Verification items for the finished model (mm, model axes). Give positions to 0.01 mm unless a question says otherwise; leave off trailing zeros. Write each loop counter-clockwise with the first axis right and the second up, starting at its lowest first coordinate (ties: lowest second). Pieces come first, ordered by that corner, then holes. Notation, with made-up numbers: (26, 60.5) -> (47, 60.5) arc R22 ccw to (47, 68.5) -> close; hole circle Ø5 at (27, -12.75). An arc over 180 degrees is marked (long way). Use one line per item in the form item = value. Start each with the question number.
(1) Section check B-B, the plane x = 0. Record the cut outline in (y, z) (1 decimal).
(2) Section check C-C, the plane y = -16.51. State how many separate pieces and enclosed holes the cut face has, plus the area to 3 significant figures.
(3) Section check A-A, the plane z = -8.89. Record the cut outline in (x, y) (3 decimals).
(4) Scan lines: L1, parallel to X at y = -7.5, z = -8.89; L2, parallel to X at y = -12.5, z = -4; L3, parallel to X at y = -10.5, z = -6.5. Record each from-to range of solid material in increasing order.
(5) Depth check by flat-ended pin: pin 1 Ø4 at (x, y) = (122.95, -16.51) entering from +Z; pin 2 Ø3 at (x, y) = (120.5, -15) entering from +Z. Enter the tip coordinate at first touch or a pass-through.
from build123d import *

# Parameters (mm, degrees)
SKETCH1_W           = 266.7
SKETCH1_H           = 17.78
SKETCH1_R           = 3.96875
BOSS_EXTRUDE1_DEPTH = 33.02
SKETCH2_R           = 3.175
CUT_EXTRUDE1_DEPTH  = 17.78
SKETCH3_R           = 4.7625
CUT_EXTRUDE2_DEPTH  = 4.7752


with BuildPart() as part:
    # Sketch1 → Boss-Extrude1 (new body)
    with BuildSketch(Plane(origin=(0, 0, 0), x_dir=(1, 0, 0), z_dir=(0, 1, 0))):
        with Locations((0, 8.89)):
            Rectangle(SKETCH1_W, SKETCH1_H)
        with Locations(Location((108.585, 8.89, 0), (0, 0, 270))):
            Circle(SKETCH1_R, mode=Mode.SUBTRACT)
        with Locations(Location((36.195, 8.89, 0), (0, 0, 270))):
            Circle(SKETCH1_R, mode=Mode.SUBTRACT)
        with Locations(Location((-36.195, 8.89, 0), (0, 0, 270))):
            Circle(SKETCH1_R, mode=Mode.SUBTRACT)
        with Locations(Location((-108.585, 8.89, 0), (0, 0, 270))):
            Circle(SKETCH1_R, mode=Mode.SUBTRACT)
    extrude(amount=-BOSS_EXTRUDE1_DEPTH)

    # Sketch2 → Cut-Extrude1 (cut)
    with BuildSketch(Plane.XY):
        with Locations((122.951875, -16.51)):
            Circle(SKETCH2_R)
        with Locations((0, -16.51)):
            Circle(SKETCH2_R)
        with Locations((-122.951875, -16.51)):
            Circle(SKETCH2_R)
    extrude(amount=-CUT_EXTRUDE1_DEPTH, mode=Mode.SUBTRACT)

    # Sketch3 → Cut-Extrude2 (cut)
    with BuildSketch(Plane.XY):
        with Locations((122.951875, -16.51)):
            Circle(SKETCH3_R)
        with Locations((0, -16.51)):
            Circle(SKETCH3_R)
        with Locations((-122.951875, -16.51)):
            Circle(SKETCH3_R)
    extrude(amount=-CUT_EXTRUDE2_DEPTH, mode=Mode.SUBTRACT)


solid = part.part
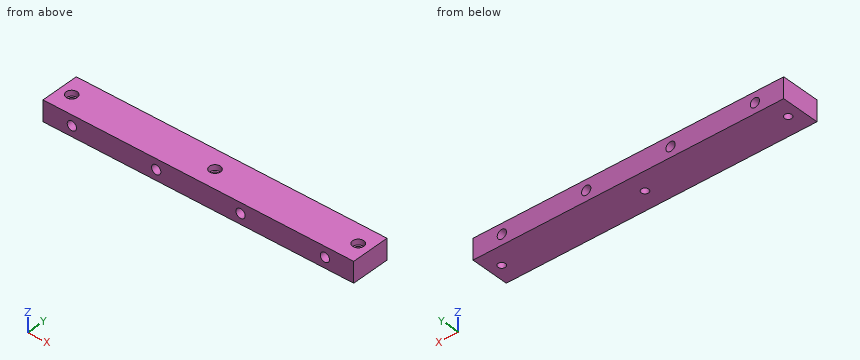
Completed:
q1.outline = (-33, -17.8) -> (-19.7, -17.8) -> (-19.7, -4.8) -> (-21.3, -4.8) -> (-21.3, 0) -> (-33, 0) -> close; (-13.3, -17.8) -> (0, -17.8) -> (0, 0) -> (-11.7, 0) -> (-11.7, -4.8) -> (-13.3, -4.8) -> close
q2.separate_pieces = 4
q2.enclosed_holes = 4
q2.area = 4,160 mm²
q3.outline = (-133.35, -33.02) -> (-112.554, -33.02) -> (-112.554, 0) -> (-133.35, 0) -> close; (-104.616, -33.02) -> (-40.164, -33.02) -> (-40.164, 0) -> (-104.616, 0) -> close; (-32.226, -33.02) -> (32.226, -33.02) -> (32.226, 0) -> (-32.226, 0) -> close; (40.164, -33.02) -> (104.616, -33.02) -> (104.616, 0) -> (40.164, 0) -> close; (112.554, -33.02) -> (133.35, -33.02) -> (133.35, 0) -> (112.554, 0) -> close; hole circle Ø6.35 at (-122.952, -16.51); hole circle Ø6.35 at (0, -16.51); hole circle Ø6.35 at (122.952, -16.51)
q4.L1 = -133.35 to -112.55, -104.62 to -40.16, -32.23 to 32.23, 40.16 to 104.62, 112.55 to 133.35
q4.L2 = -133.35 to -125.52, -120.38 to -2.57, 2.57 to 120.38, 125.52 to 133.35
q4.L3 = -133.35 to -111.75, -105.42 to -39.36, -33.03 to 33.03, 39.36 to 105.42, 111.75 to 133.35
q5.pin_1 = through
q5.pin_2 = -4.78
